from build123d import *

# Parameters (mm, degrees)
BOSS_EXTRUDE1_DEPTH = 30
SKETCH4_W           = 16
SKETCH4_H           = 14
CUT_EXTRUDE2_DEPTH  = 25
SKETCH5_W           = 5.5
SKETCH5_H           = 1.8
CUT_EXTRUDE3_DEPTH  = 15
CUT_EXTRUDE4_DEPTH  = 11.5
BOSS_EXTRUDE2_DEPTH = 8
SKETCH8_W           = 4.5
SKETCH8_H           = 9.4
CUT_EXTRUDE5_DEPTH  = 47.486557197
SKETCH9_W           = 5.5
SKETCH9_H           = 1.8
CUT_EXTRUDE6_DEPTH  = 47.486557197


with BuildPart() as part:
    # Sketch1 → Boss-Extrude1 (new body)
    with BuildSketch(Plane.XY):
        Polygon((0, 0), (0, -30), (12, -30), (12, -20), (5, 0), align=None)
    extrude(amount=-BOSS_EXTRUDE1_DEPTH)

    # Sketch4 → Cut-Extrude2 (cut)
    with BuildSketch(Plane.ZY):
        with Locations((-15, -23.917856259)):
            Rectangle(SKETCH4_W, SKETCH4_H)
    extrude(amount=-CUT_EXTRUDE2_DEPTH, mode=Mode.SUBTRACT)

    # Sketch5 → Cut-Extrude3 (cut)
    with BuildSketch(Plane.ZY):
        with Locations((-4.25, -27.7)):
            Rectangle(SKETCH5_W, SKETCH5_H)
    extrude(amount=-CUT_EXTRUDE3_DEPTH, mode=Mode.SUBTRACT)

    # Sketch6 → Cut-Extrude4 (cut, symmetric)
    with BuildSketch(Plane.XY.offset(-15.5)):
        Polygon((5, 0), (5, -14), (9.9, -14), align=None)
    extrude(amount=CUT_EXTRUDE4_DEPTH, both=True, mode=Mode.SUBTRACT)

    # Sketch7 → Boss-Extrude2 (add)
    with BuildSketch(Plane(origin=(0, -22, 0), x_dir=(1, 0, 0), z_dir=(0, 1, 0))):
        with BuildLine():
            Line((0, 27.7), (-19, 27.7))
            Line((-19, 27.7), (-19, 26.2))
            Line((-19, 26.2), (-16.993455994, 26.2))
            ThreePointArc((-16.993455994, 26.2), (-16.6644108, 25.067952934), (-16.365476207, 23.927584833))
            Line((-16.365476207, 23.927584833), (-15.609396851, 24.115112691))
            Line((-15.609396851, 24.115112691), (-15.179008189, 26.2))
            Line((-15.179008189, 26.2), (-14.896454824, 26.2))
            ThreePointArc((-14.896454824, 26.2), (-14.56740963, 25.067952934), (-14.268475038, 23.927584833))
            Line((-14.268475038, 23.927584833), (-13.512395681, 24.115112691))
            Line((-13.512395681, 24.115112691), (-13.082007019, 26.2))
            Line((-13.082007019, 26.2), (-12.799453654, 26.2))
            ThreePointArc((-12.799453654, 26.2), (-12.470408461, 25.067952934), (-12.171473868, 23.927584833))
            Line((-12.171473868, 23.927584833), (-11.415394512, 24.115112691))
            Line((-11.415394512, 24.115112691), (-10.985005849, 26.2))
            Line((-10.985005849, 26.2), (-10.702452484, 26.2))
            ThreePointArc((-10.702452484, 26.2), (-10.373407291, 25.067952934), (-10.074472698, 23.927584833))
            Line((-10.074472698, 23.927584833), (-9.318393342, 24.115112691))
            Line((-9.318393342, 24.115112691), (-8.888004679, 26.2))
            Line((-8.888004679, 26.2), (-8.605451315, 26.2))
            ThreePointArc((-8.605451315, 26.2), (-8.276406121, 25.067952934), (-7.977471528, 23.927584833))
            Line((-7.977471528, 23.927584833), (-7.221392172, 24.115112691))
            Line((-7.221392172, 24.115112691), (-6.791003509, 26.2))
            Line((-6.791003509, 26.2), (-6.508450145, 26.2))
            ThreePointArc((-6.508450145, 26.2), (-6.179404951, 25.067952934), (-5.880470358, 23.927584833))
            Line((-5.880470358, 23.927584833), (-5.124391002, 24.115112691))
            Line((-5.124391002, 24.115112691), (-4.69400234, 26.2))
            Line((-4.69400234, 26.2), (-4.411448975, 26.2))
            ThreePointArc((-4.411448975, 26.2), (-4.082403781, 25.067952934), (-3.783469189, 23.927584833))
            Line((-3.783469189, 23.927584833), (-3.027389832, 24.115112691))
            Line((-3.027389832, 24.115112691), (-2.59700117, 26.2))
            Line((-2.59700117, 26.2), (-2.314447805, 26.2))
            ThreePointArc((-2.314447805, 26.2), (-1.985402612, 25.067952934), (-1.686468019, 23.927584833))
            Line((-1.686468019, 23.927584833), (-0.930388662, 24.115112691))
            Line((-0.930388662, 24.115112691), (-0.5, 26.2))
            Line((-0.5, 26.2), (0, 26.2))
            Line((0, 26.2), (0, 27.7))
        make_face()
    extrude(amount=BOSS_EXTRUDE2_DEPTH)

    # Sketch8 → Cut-Extrude5 (cut, through all)
    with BuildSketch(Plane.ZY):
        with Locations((-4.168450475, -18.374722701)):
            Rectangle(SKETCH8_W, SKETCH8_H)
    extrude(amount=-CUT_EXTRUDE5_DEPTH, mode=Mode.SUBTRACT)

    # Sketch9 → Cut-Extrude6 (cut, through all)
    with BuildSketch(Plane.ZY):
        with Locations((-25.635290025, -27.453702253)):
            Rectangle(SKETCH9_W, SKETCH9_H)
    extrude(amount=-CUT_EXTRUDE6_DEPTH, mode=Mode.SUBTRACT)


solid = part.part
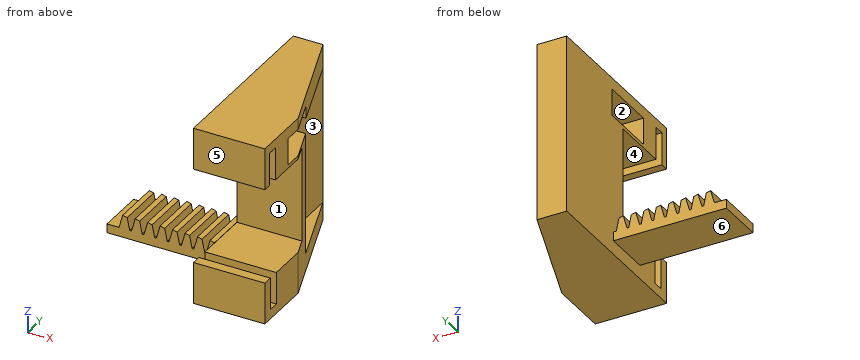
Part model, mm, in its own coordinate system. Face numbers are marked on the shaded views. A direction names the side the tool comes from. Round coordinates to 2 decimals unless told otherwise and drop trailing zeros. Loops run counter-clockwise (first coordinate to the right, second up) from the corner with the lowest first, then second, coordinate; pieces in that order, holes last. Notation, with made-up numbers: (28, -1.75) - (54, -1.75) arc R8 ccw to (54, 8.25) - close; hole circle Ø3 at (25.5, 79.5). An arc over 180 degrees is marked (long way). Answer as a JSON object with one key per item and string values.
Item 1: Band-saw the part on D-D on y = -9. List the corners of the cut face in (x, z), plus the area to 3 significant figures.
Output:
{"outline": "(0, -30) - (8.15, -30) - (8.15, -27) - (5, -27) - (5, -4) - (8.15, -4) - (8.15, 0) - (0, 0) - close", "area": "172 mm2"}
Item 2: Pin check, flat tips, straight feed: pin 1 (1.5 mm diameter, centred on y = -4.5, z = -12, fed in from +X); pin 2 (3 mm diameter, centred on x = -6, y = -11.5, fed in from -Z); pin 3 (4.5 mm diameter, centred on x = 4.5, z = -26, fed in from +Y); pin 4 (3 mm diameter, centred on x = -8, z = -26.5, fed in from +Y). Stop position of each tip, or through.
Output:
{"pin 1": "x = 5", "pin 2": "through", "pin 3": "y = 0", "pin 4": "y = -14"}
Item 3: Tool access for the marked faces 1, 2 and 3: list every direction of +Z, -Z, +X, -X, +Y, -Y with a clear straight run to the whole face (end or side of a thin tool).
Output:
{"face 1": "+X, -X, -Y", "face 2": "+X, -X", "face 3": "+X, +Y"}
Item 4: Band-saw the part on C-C on z = -5.5. List the corners of the cut face in (x, y), plus the area to 3 significant figures.
Output:
{"outline": "(0, -30) - (12, -30) - (12, -28.6) - (0, -28.6) - close; (0, -26.8) - (12, -26.8) - (12, -23.07) - (0, -23.07) - close; (0, -13.67) - (5, -13.67) - (5, 0) - (0, 0) - close", "area": "130 mm2"}
Item 5: Band-saw the part on A-A on y = -25. List the corners of the cut face in (x, z), plus the area to 3 significant figures.
Output:
{"outline": "(0, -30) - (12, -30) - (12, -23) - (0, -23) - close; (0, -7) - (12, -7) - (12, 0) - (0, 0) - close", "area": "168 mm2"}
Item 6: Wall check: L1, parallel to Z at x = 10, y = -20.5; L2, parallel to Y at x = 9, z = -6; L3, parallel to Y at x = 4.5, z = -23.5. Give the ranges that are in metal, low to high.
Output:
{"L1": "-30 to -23, -7 to -6.42, -1.92 to 0", "L2": "-30 to -28.6, -26.8 to -23.07", "L3": "-30 to -28.35, -26.55 to 0"}
Item 7: Pull direction Z, two halves, no side cores. Call the marked faces 4, 5 and 6: pulls with the +Z half, pulls with the -Z half, needs draft (parallel to the pull), parting line crosses it, or undercut.
Output:
{"face 4": "undercut", "face 5": "needs draft", "face 6": "pulls with the -Z half"}
Item 8: Band-saw the part on B-B on x = 4. List the corners of the cut face in (y, z).
Output:
{"outline": "(-30, -30) - (0, -30) - (0, 0) - (-30, 0) - (-30, -7) - (-28.6, -7) - (-28.6, -1.5) - (-26.8, -1.5) - (-26.8, -7) - (-16.92, -7) - (-16.92, -23) - (-26.55, -23) - (-26.55, -28.39) - (-28.35, -28.39) - (-28.35, -23) - (-30, -23) - close; hole (-23.07, -6.42) - (-13.67, -6.42) - (-13.67, -1.92) - (-23.07, -1.92) - close"}
